Read the model definition and answer for the solid it produces. Units are mm, in the model's axes. Coordinates: 2 decimals unless noted, no trailing zeros. Write each loop counter-clockwise with the first axis right and the second up, starting at its lowest first coordinate (ties: lowest second). Pieces come first, ordered by that corner, then holes.
Item 1: Section C-C (y = 2.5) is taken. Give the vertices of the cut face in (x, z).
Item 2: Each of these flat-tipped pins is pushed along its axis until it touches: P1, Ø1, axis at x = 13.5, z = 3, coming from the -Y side; P2, Ø3, axis at x = 6, y = 14.5, coming from the +Z side; P3, Ø2, axis at x = 10, y = 3, coming from the +Z side. Where does it stop, or does it pass through?
Item 3: Straight lines are drawn through the part: probe 1 along Z at (x, y) = (6, 1.5); probe 2 along X at (y, z) = (11, 2.75); probe 3 along X at (y, z) = (12, 4.75). For each, find the intervals that lie inside material, in ascending order.
Item 4: Section B-B (x = 1.25) is taken. Give the vertices of the cut face in (y, z), then the cut area to 3 significant figures.
Item 5: Determine the mould class of faces 1 (the face through (9.05, 10.43, 4.74)), 2 (the face through (16, 11, 1)), 3 (the face through (7.9, 14.2, 2)), 4 (the face through (8, 12, 0)) for opening direction Z: released by +Z, released by -Z, zero draft, split by the parting line, or undercut.
Item 6: Section A-A (z = 6) is taken. Give the vertices of the cut face in (x, y), then the cut area to 3 significant figures.
from build123d import *

# Parameters (mm, degrees)
SKETCH1_W           = 16
SKETCH1_H           = 23
BOSS_EXTRUDE1_DEPTH = 2
SKETCH6_R           = 1.5
BOSS_EXTRUDE3_DEPTH = 1.5
SKETCH7_R           = 1.5
BOSS_EXTRUDE4_DEPTH = 1
BOSS_EXTRUDE4_DRAFT = -20


with BuildPart() as part:
    # Sketch1 → Boss-Extrude1 (new body)
    with BuildSketch(Plane.XY):
        with Locations((8, 11.5)):
            Rectangle(SKETCH1_W, SKETCH1_H)
    extrude(amount=BOSS_EXTRUDE1_DEPTH)

    # Loft1: read off the stored shape, not the designer's step
    # Loft1: loft between two sections, ruled curve by curve
    loft1_from = [
        Edge.make_bspline([(10.5, 11.5, 2), (10.5, 16.5, 2), (5.5, 16.5, 2), (5.5, 11.5, 2), (5.5, 6.5, 2), (10.5, 6.5, 2), (10.5, 11.5, 2)], [0, 0, 0, 0, 0.5, 0.5, 0.5, 1, 1, 1, 1], 3, [1, 0.333333333, 0.333333333, 1, 0.333333333, 0.333333333, 1]),
    ]
    loft1_to = [
        Edge.make_bspline([(9.382185261, 10.91727888, 4), (10.547627501, 13.681649403, 4), (7.783256979, 14.847091642, 4), (6.617814739, 12.08272112, 4), (5.452372499, 9.318350597, 4), (8.216743021, 8.152908358, 4), (9.382185261, 10.91727888, 4)], [0, 0, 0, 0, 0.5, 0.5, 0.5, 1, 1, 1, 1], 3, [1, 0.333333333, 0.333333333, 1, 0.333333333, 0.333333333, 1]),
    ]
    loft1 = Solid(Shell([*[Face.make_surface_from_curves(loft1_from[k], loft1_to[k]) for k in range(1)], Face(Wire(loft1_from)), Face(Wire(loft1_to))]))
    add(loft1)

    # Sketch6 → Boss-Extrude3 (add)
    with BuildSketch(Plane.XY.offset(4)):
        with Locations(Location((8, 11.5, 0), (0, 0, 337.14))):
            Circle(SKETCH6_R)
    extrude(amount=BOSS_EXTRUDE3_DEPTH)


with BuildPart() as boss_extrude4_tool:
    # Sketch7 → Boss-Extrude4 (with draft: the straight prism first)
    with BuildSketch(Plane.XY.offset(5.5)):
        with Locations(Location((8, 11.5, 0), (0, 0, 337.14))):
            Circle(SKETCH7_R)
    extrude(amount=BOSS_EXTRUDE4_DEPTH)
    # Boss-Extrude4: the draft: its side faces are tilted about the plane it starts from
    boss_extrude4_sides = [boss_extrude4_tool.faces().sort_by_distance(p)[0] for p in [
        (6.617814739, 12.08272112, 6),
    ]]
    draft(boss_extrude4_sides, Plane.XY.offset(5.5), BOSS_EXTRUDE4_DRAFT)


with BuildPart() as part_1:
    add(part.part)

    # Boss-Extrude4: add boss_extrude4_tool
    add(boss_extrude4_tool.part)


solid = part_1.part
Established:
1. outline: (0, 0) - (16, 0) - (16, 2) - (0, 2) - close
2. P1: passes through
2. P2: stops at z = 2.72
2. P3: stops at z = 2
3. probe 1: z = 0 to 2
3. probe 2: x = 5.97 to 10.03
3. probe 3: x = 6.59 to 9.41
4. outline: (0, 0) - (23, 0) - (23, 2) - (0, 2) - close
4. area: 46.0 mm2
5. face 1: undercut
5. face 2: zero draft
5. face 3: released by +Z
5. face 4: released by -Z
6. outline: circle Ø3.36 at (8, 11.5)
6. area: 8.89 mm2
